Build history of the part. All positions in model axes, mm. A direction names the side the tool comes from. Give positions to 0.01 mm unless a question says otherwise; leave off trailing zeros. Loops run counter-clockwise (first coordinate to the right, second up) from the corner with the lowest first, then second, coordinate; pieces in that order, holes last.
1) Flat gauge pins, fed straight in: P1, Ø1, axis at y = -6.5, z = 3.5, coming from the +X side; P2, Ø1.5, axis at x = 31, z = 3, coming from the +Y side; P3, Ø8, axis at x = -2.5, y = -145, coming from the -Z side; P4, Ø1.5, axis at y = -20.5, z = 2.5, coming from the -X side. Where does each tip first touch, or does it go through?
2) 3-axis set-ups, long thin cutter, end or side, ignore diameter. For faces 1 (the flat face through (-16, -94, 0)), 2 (the flat face through (32, -105.038, 3)): which of +Z, -Z, +X, -X, +Y, -Y reach the whole face in a straight line?
3) Band-saw the part on C-C on y = -28.5. List the corners of the cut face in (x, z).
4) Band-saw the part on D-D on x = -27. List the corners of the cut face in (y, z), then the cut area to 3 significant figures.
5) Band-saw the part on A-A on y = -160. List the corners of the cut face in (x, z).
6) Wall check: line 1 (X direction, y = -18, z = 2.7); line 2 (X direction, y = -107, z = 4.1); line 3 (Y direction, x = -2, z = 2.15). Give the ranges that are in metal, low to high.
7) Band-saw the part on B-B on z = 3.8. State how many separate pieces and enclosed holes the cut face has, then the cut area to 3 significant figures.
8) Two-plate mould, pull along X, no slides. Class faces 3 (the flat face through (27.32, 6.67, 2.46)), 4 (the cylindrical face through (-81.27, -158.23, 2.54)), 5 (the flat face through (32, -100.038, 3)), 6 (the flat face through (-112.4, -128, 3)): +X half, -X half, draft (parallel to the pull), parting line (faces both ways), or undercut.
```python
from build123d import *
from build123d.topology import SkipClean

# Parameters (mm, degrees)
SKETCH_1_R          = 2.6
SKETCH_1_R_2        = 4.1
EXTRUDE_1_DEPTH     = 5
SKETCH_2_R          = 13.5
SKETCH_2_R_2        = 1.6
EXTRUDE_2_DEPTH     = 5
CUT_EXTRUDE_START   = -10
SKETCH_3_R          = 2.6
CUT_EXTRUDE_1_DEPTH = 10
CUT_EXTRUDE_3_DEPTH = 5
SKETCH_6_R          = 1.5
CUT_EXTRUDE_5_DEPTH = 204.859657608
SKETCH_7_W          = 14.99904054
SKETCH_7_H          = 5
CUT_EXTRUDE_6_DEPTH = 204.859657608
SKETCH_8_W          = 64.8
SKETCH_8_H          = 20
EXTRUDE_3_DEPTH     = 5
SKETCH_9_R          = 2.1
CUT_EXTRUDE_7_DEPTH = 5


with BuildPart() as part:
    # 草图1 → 凸台-拉伸1 (new body)
    with BuildSketch(Plane.XY):
        with BuildLine():
            Line((-42.831, 7.053044662), (-8.38125, 20.880724327))
            ThreePointArc((-8.38125, 20.880724327), (0, 22.5), (8.38125, 20.880724327))
            Line((8.38125, 20.880724327), (42.831, 7.053044662))
            ThreePointArc((42.831, 7.053044662), (46.29585578, 4.257017735), (47.6, 0))
            Line((47.6, 0), (47.6, -170))
            Line((47.6, -170), (-47.6, -170))
            Line((-47.6, -170), (-47.6, 0))
            ThreePointArc((-47.6, 0), (-46.29585578, 4.257017735), (-42.831, 7.053044662))
        make_face()
        with Locations((-40, 0)):
            Circle(SKETCH_1_R, mode=Mode.SUBTRACT)
        with Locations(Location((40, 0, 0), (0, 0, 180))):
            Circle(SKETCH_1_R, mode=Mode.SUBTRACT)
        Circle(SKETCH_1_R_2, mode=Mode.SUBTRACT)
    extrude(amount=EXTRUDE_1_DEPTH)

    # 草图2 → 凸台-拉伸2 (add)
    with BuildSketch(Plane.XY.offset(5)):
        Polygon((-47.6, -47.587702557), (-47.6, -150), (-112.4, -150), (-112.4, -85), align=None)
        with Locations((-81.662414855, -107.5)):
            Circle(SKETCH_2_R, mode=Mode.SUBTRACT)
        with Locations((-81.662414855, -90)):
            Circle(SKETCH_2_R_2, mode=Mode.SUBTRACT)
        with Locations((-64.162414855, -107.5)):
            Circle(SKETCH_2_R_2, mode=Mode.SUBTRACT)
        with Locations((-81.662414855, -125)):
            Circle(SKETCH_2_R_2, mode=Mode.SUBTRACT)
        with Locations((-99.162414855, -107.5)):
            Circle(SKETCH_2_R_2, mode=Mode.SUBTRACT)
    extrude(amount=-EXTRUDE_2_DEPTH)

    # 草图3 → 切除-拉伸1 (cut)
    with SkipClean():  # the faces are left unmerged after this step: merging them gives an invalid solid
        with BuildSketch(Plane.XY.offset(5).offset(CUT_EXTRUDE_START)):
            with Locations((0, 18)):
                Circle(SKETCH_3_R)
            with Locations((0, -18)):
                Circle(SKETCH_3_R)
            with BuildLine():
                Line((-14.287145834, 17.381814172), (-47.6, -10))
                Line((-47.6, -10), (-95.969286822, 101.060273712))
                Line((-95.969286822, 101.060273712), (-90.307154963, 103.526261511))
                Line((-90.307154963, 103.526261511), (99.481091757, 68.842428386))
                Line((99.481091757, 68.842428386), (47.6, -10))
                Line((47.6, -10), (14.287145834, 17.381814172))
                ThreePointArc((14.287145834, 17.381814172), (0, 22.5), (-14.287145834, 17.381814172))
            make_face()
        extrude(amount=CUT_EXTRUDE_1_DEPTH, mode=Mode.SUBTRACT)

    # 草图5 → 切除-拉伸3 (cut)
    with SkipClean():  # the faces are left unmerged after this step: merging them gives an invalid solid
        with BuildSketch(Plane.XY.offset(5)):
            Polygon((40, -3.753108435), (47.6, -16.916694572), (47.6, -10), align=None)
        extrude(amount=-CUT_EXTRUDE_3_DEPTH, mode=Mode.SUBTRACT)

    # 草图6 → 切除-拉伸5 (cut, through all)
    with SkipClean():  # the faces are left unmerged after this step: merging them gives an invalid solid
        with BuildSketch(Plane.XY.offset(5)):
            with Locations((1.5, -105)):
                Circle(SKETCH_6_R)
            with Locations((1.5, -100)):
                Circle(SKETCH_6_R)
            with Locations((13.5, -105)):
                Circle(SKETCH_6_R)
            with Locations((13.5, -100)):
                Circle(SKETCH_6_R)
            with Locations((38.1, -105)):
                Circle(SKETCH_6_R)
            with Locations((26.1, -105)):
                Circle(SKETCH_6_R)
            with Locations((26.1, -100)):
                Circle(SKETCH_6_R)
            with Locations((38.1, -100)):
                Circle(SKETCH_6_R)
        extrude(amount=-CUT_EXTRUDE_5_DEPTH, mode=Mode.SUBTRACT)

    # 草图7 → 切除-拉伸6 (cut, through all)
    with SkipClean():  # the faces are left unmerged after this step: merging them gives an invalid solid
        with BuildSketch(Plane.XY.offset(5)):
            with Locations((7.5, -102.537933644)):
                Rectangle(SKETCH_7_W, SKETCH_7_H)
            with Locations((32.1, -102.537933644)):
                Rectangle(SKETCH_7_W, SKETCH_7_H)
        extrude(amount=-CUT_EXTRUDE_6_DEPTH, mode=Mode.SUBTRACT)

    # 草图8 → 凸台-拉伸3 (add)
    with SkipClean():  # the faces are left unmerged after this step: merging them gives an invalid solid
        with BuildSketch(Plane.XY.offset(5)):
            with Locations((-80, -160)):
                Rectangle(SKETCH_8_W, SKETCH_8_H)
        extrude(amount=-EXTRUDE_3_DEPTH)

    # 草图9 → 切除-拉伸7 (cut)
    with SkipClean():  # the faces are left unmerged after this step: merging them gives an invalid solid
        with BuildSketch(Plane.XY.offset(5)):
            with Locations((-102.4, -160)):
                Circle(SKETCH_9_R)
            with Locations((-82.4, -160)):
                Circle(SKETCH_9_R)
            with Locations((-62.4, -160)):
                Circle(SKETCH_9_R)
            with Locations(Location((-2.4, -160, 0), (0, 0, 180))):
                Circle(SKETCH_9_R)
            with Locations(Location((17.6, -160, 0), (0, 0, 180))):
                Circle(SKETCH_9_R)
            with Locations(Location((37.6, -160, 0), (0, 0, 180))):
                Circle(SKETCH_9_R)
        extrude(amount=-CUT_EXTRUDE_7_DEPTH, mode=Mode.SUBTRACT)


solid = part.part
```
Findings below:
1. P1: stops at x = 41.87
1. P2: stops at y = 4.26
1. P3: stops at z = 0
1. P4: stops at x = -47.6
2. face 1: -Z, +X, -X, +Y, -Y
2. face 2: +Z, -Z
3. outline: (-47.6, 0) - (47.6, 0) - (47.6, 5) - (-47.6, 5) - close
4. outline: (-170, 0) - (6.93, 0) - (6.93, 5) - (-170, 5) - close
4. area: 885 mm2
5. outline: (-112.4, 0) - (-104.5, 0) - (-104.5, 5) - (-112.4, 5) - close; (-100.3, 0) - (-84.5, 0) - (-84.5, 5) - (-100.3, 5) - close; (-80.3, 0) - (-64.5, 0) - (-64.5, 5) - (-80.3, 5) - close; (-60.3, 0) - (-4.5, 0) - (-4.5, 5) - (-60.3, 5) - close; (-0.3, 0) - (15.5, 0) - (15.5, 5) - (-0.3, 5) - close; (19.7, 0) - (35.5, 0) - (35.5, 5) - (19.7, 5) - close; (39.7, 0) - (47.6, 0) - (47.6, 5) - (39.7, 5) - close
6. line 1: x = -47.6 to -2.6, 2.6 to 47.6
6. line 2: x = -112.4 to -100.68, -97.64 to -95.15, -68.17 to -65.68, -62.64 to 47.6
6. line 3: y = -170 to -162.06, -157.94 to -19.66, -16.34 to -3.58, 3.58 to 16.34, 19.66 to 22.41
7. separate pieces: 1
7. enclosed holes: 16
7. area: 22,800 mm2
8. face 3: +X half
8. face 4: undercut
8. face 5: undercut
8. face 6: -X half
